Part model, mm, in its own coordinate system. Coordinates: 2 decimals unless noted, no trailing zeros. Loops run counter-clockwise (first coordinate to the right, second up) from the corner with the lowest first, then second, coordinate; pieces in that order, holes last.
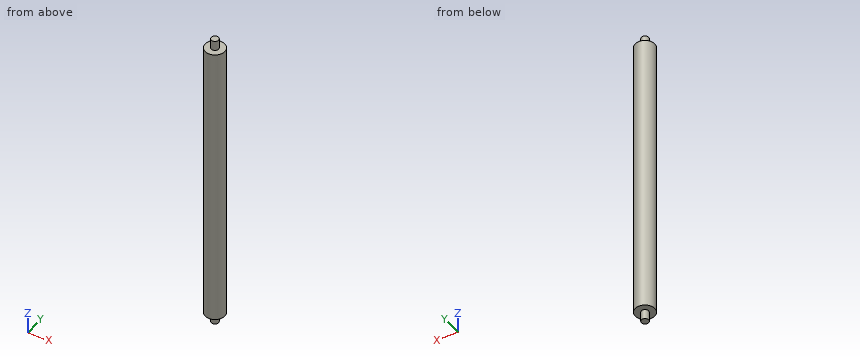
```python
from build123d import *

# Parameters (mm, degrees)
SKETCH_1_R      = 4
EXTRUDE_1_DEPTH = 118
SKETCH_2_R      = 1.5
EXTRUDE_2_DEPTH = 4
SKETCH_3_R      = 1.5
EXTRUDE_3_DEPTH = 4


with BuildPart() as part:
    # 草图1 → 凸台-拉伸1 (new body)
    with BuildSketch(Plane.XY):
        Circle(SKETCH_1_R)
    extrude(amount=EXTRUDE_1_DEPTH)

    # 草图2 → 凸台-拉伸2 (add)
    with BuildSketch(Plane(origin=(0, 0, 0), x_dir=(-1, 0, 0), z_dir=(0, 0, -1))):
        Circle(SKETCH_2_R)
    extrude(amount=EXTRUDE_2_DEPTH)

    # 草图3 → 凸台-拉伸3 (add)
    with BuildSketch(Plane.XY.offset(118)):
        Circle(SKETCH_3_R)
    extrude(amount=EXTRUDE_3_DEPTH)


solid = part.part
```
Q1. Saw through at A-A (x = 0). List the corners of the cut face in (y, z).
Q2. Saw through at C-C (z = 41). List the corners of the cut face in (x, y), plus the area to 3 significant figures.
Q3. Probe line 1 (Z direction, x = 0.5, y = -2.5); line 2 (X direction, y = 0.25, z = 6); line 3 (Y direction, x = -2, z = 103). List the from-to ranges inside material, lowest first.
Q4. Drop flat-ended pins along their axis: P1, Ø3, axis at x = 3, y = -2.5, coming from the -Z side; P2, Ø1.5, axis at y = 2.5, z = 19.5, coming from the -X side; P3, Ø1.5, axis at y = -1, z = 88, coming from the -X side. Give the stop position or say it passes through.
Checked values:
1. outline: (-4, 0) - (-1.5, 0) - (-1.5, -4) - (1.5, -4) - (1.5, 0) - (4, 0) - (4, 118) - (1.5, 118) - (1.5, 122) - (-1.5, 122) - (-1.5, 118) - (-4, 118) - close
2. outline: circle Ø8 at (0, 0)
2. area: 50.3 mm2
3. line 1: z = 0 to 118
3. line 2: x = -3.99 to 3.99
3. line 3: y = -3.46 to 3.46
4. P1: stops at z = 0
4. P2: stops at x = -3.6
4. P3: stops at x = -3.99
